```python
from build123d import *

# Parameters (mm, degrees)
BOSS_EXTRUDE1_DEPTH = 20
CUT_EXTRUDE1_REACH  = 38.702
SKETCH2_R           = 2.5
SKETCH5_W           = 10
SKETCH5_H           = 18
CUT_EXTRUDE4_DEPTH  = 54.272627403
SKETCH6_R           = 4
CUT_EXTRUDE5_DEPTH  = 46.762260698
SKETCH8_W           = 6
SKETCH8_H           = 22.840741565
CUT_EXTRUDE6_DEPTH  = 37.702076275
SKETCH12_W          = 3.539135452
SKETCH12_H          = 18
CUT_EXTRUDE7_DEPTH  = 41.024339686
CUT_EXTRUDE8_REACH  = 39.827
SKETCH13_W          = 12
SKETCH13_H          = 14.840741565
FILLET2_R           = 0.5


with BuildPart() as part:
    # Sketch1 → Boss-Extrude1 (new body)
    with BuildSketch(Plane.XY):
        Polygon((-3.287943452, 12.452372753), (-3.287943452, -24.388368812), (6.712056548, -24.388368812), (6.712056548, 17.547627247), (11.11006124, 19.788522565), (6.570156243, 28.698587807), (-7.827848449, 21.362437994), align=None)
    extrude(amount=BOSS_EXTRUDE1_DEPTH)

    # Sketch2 → Cut-Extrude1 (cut, up to next)
    with BuildSketch(Plane(origin=(0, 0, 0), x_dir=(-1, 0, 0), z_dir=(0, 0, -1)), mode=Mode.PRIVATE) as cut_extrude1_sk1:
        with Locations((-1.712056548, -19.388368812)):
            Circle(SKETCH2_R)
    cut_extrude1_tool1 = extrude(cut_extrude1_sk1.sketch, amount=-CUT_EXTRUDE1_REACH, mode=Mode.PRIVATE) & part.part
    # Sketch2 → Cut-Extrude1 (cut, up to next)
    with BuildSketch(Plane(origin=(0, 0, 0), x_dir=(-1, 0, 0), z_dir=(0, 0, -1)), mode=Mode.PRIVATE) as cut_extrude1_sk2:
        with Locations((-1.712056548, 20.611631188)):
            Circle(SKETCH2_R)
    cut_extrude1_tool2 = extrude(cut_extrude1_sk2.sketch, amount=-CUT_EXTRUDE1_REACH, mode=Mode.PRIVATE) & part.part
    add(cut_extrude1_tool1.solids().sort_by_distance((1.712057, -19.388369, 0))[0], mode=Mode.SUBTRACT)
    add(cut_extrude1_tool2.solids().sort_by_distance((1.712057, 20.611631, 0))[0], mode=Mode.SUBTRACT)

    # Sketch5 → Cut-Extrude4 (cut, through all)
    with BuildSketch(Plane(origin=(-10.254664976, 20.125913213, 0), x_dir=(0.891006524188368, 0.4539904997395467, 0), z_dir=(-0.4539904997395467, 0.891006524188368, 0))):
        with Locations((10.843123689, -10)):
            Rectangle(SKETCH5_W, SKETCH5_H)
    extrude(amount=-CUT_EXTRUDE4_DEPTH, mode=Mode.SUBTRACT)

    # Sketch6 → Cut-Extrude5 (cut, through all)
    with BuildSketch(Plane(origin=(16.824821219, 8.572674594, 0), x_dir=(0, 0, -1), z_dir=(0.891006524188368, 0.45399049973954647, 0))):
        with Locations(Location((-10, 17.587840455, 0), (0, 0, 90))):
            Circle(SKETCH6_R)
    extrude(amount=-CUT_EXTRUDE5_DEPTH, mode=Mode.SUBTRACT)

    # Sketch8 → Cut-Extrude6 (cut, through all)
    with BuildSketch(Plane.XY.offset(20)):
        with Locations((1.712056548, -2.96799803)):
            Rectangle(SKETCH8_W, SKETCH8_H)
    extrude(amount=-CUT_EXTRUDE6_DEPTH, mode=Mode.SUBTRACT)

    # Sketch12 → Cut-Extrude7 (cut, through all)
    with BuildSketch(Plane.XZ.offset(-8.452372753)):
        with Locations((0.481624274, 10)):
            Rectangle(SKETCH12_W, SKETCH12_H)
    extrude(amount=-CUT_EXTRUDE7_DEPTH, mode=Mode.SUBTRACT)

    # Sketch13 → Cut-Extrude8 (cut, up to next)
    with BuildSketch(Plane.ZY.offset(3.287943452), mode=Mode.PRIVATE) as cut_extrude8_sk1:
        with Locations((10, -6.96799803)):
            Rectangle(SKETCH13_W, SKETCH13_H)
    cut_extrude8_tool1 = extrude(cut_extrude8_sk1.sketch, amount=-CUT_EXTRUDE8_REACH, mode=Mode.PRIVATE) & part.part
    add(cut_extrude8_tool1.solids().sort_by_distance((-3.287943, -6.967998, 10))[0], mode=Mode.SUBTRACT)

    # Fillet2
    fillet2_edges = [part.edges().sort_by_distance(p)[0] for p in [
        (-2.287943452, -14.388368812, 4),
        (-1.287943452, -14.388368812, 18),
        (-1.287943452, -14.388368812, 2),
        (4.712056548, -14.388368812, 10),
        (-1.287943452, -6.96799803, 4),
        (-2.287943452, 0.452372753, 4),
        (-1.287943452, 0.452372753, 10),
        (-2.287943452, 0.452372753, 16),
        (-2.287943452, -14.388368812, 16),
        (-1.287943452, -6.96799803, 16),
        (1.712056548, 8.452372753, 19),
        (1.712056548, 8.452372753, 0),
        (1.712056548, 8.452372753, 1),
        (4.712056548, -2.96799803, 0),
        (-1.287943452, -2.96799803, 0),
        (1.712056548, -14.388368812, 0),
        (1.712056548, 8.452372753, 20),
        (4.712056548, -2.96799803, 20),
        (1.712056548, -14.388368812, 20),
        (-1.287943452, -2.96799803, 20),
        (-3.287943452, -14.388368812, 10),
        (-3.287943452, -6.96799803, 4),
        (-3.287943452, 0.452372753, 10),
        (-3.287943452, -6.96799803, 16),
        (1.712056548, -24.388368812, 20),
        (1.712056548, -24.388368812, 0),
        (-3.287943452, -24.388368812, 10),
        (-3.287943452, -5.96799803, 20),
        (-5.55789595, 16.907405373, 20),
        (-3.287943452, 12.452372753, 10),
        (-5.55789595, 16.907405373, 0),
        (-3.287943452, -5.96799803, 0),
        (-0.628846103, 25.030512901, 20),
        (-0.593371027, 25.048588355, 19),
        (-5.048403648, 22.778635856, 10),
        (-7.827848449, 21.362437994, 10),
        (-0.628846103, 25.030512901, 0),
        (-0.593371027, 25.048588355, 1),
        (3.861661594, 27.318540854, 10),
        (6.570156243, 28.698587807, 10),
        (8.840108742, 24.243555186, 20),
        (8.840108742, 24.243555186, 0),
        (11.11006124, 19.788522565, 10),
        (7.55681157, 17.97805143, 19),
        (8.911058894, 18.668074906, 20),
        (7.55681157, 17.97805143, 1),
        (8.401566592, 18.408475612, 10),
        (6.712056548, 8.622530187, 1),
        (4.712056548, 6.037513445, 19),
        (6.712056548, 8.622530187, 19),
        (4.712056548, 3.622654137, 10),
        (6.712056548, -0.302566874, 10),
        (8.911058894, 18.668074906, 0),
        (6.712056548, -3.420370782, 0),
        (6.712056548, -24.388368812, 10),
        (6.712056548, -3.420370782, 20),
    ]]
    fillet(fillet2_edges, radius=FILLET2_R - 0.0001)  # a hair under: the kernel refuses the full size


solid = part.part
```
Work out the finished part from the listing and answer in its coordinate system (mm). A direction names the side the tool comes from. Give positions to 0.01 mm unless a question says otherwise; leave off trailing zeros. Write each loop counter-clockwise with the first axis right and the second up, starting at its lowest first coordinate (ties: lowest second). Pieces come first, ordered by that corner, then holes. Notation, with made-up numbers: (69.5, 23) - (86.5, 23) arc R33 ccw to (86.5, 62) - close; hole circle Ø7 at (33, -15). An arc over 180 degrees is marked (long way). Use one line per item in the form item = value.
1. A cutting plane is placed at C-C (y = -16). Write down the section's boundary in (x, z), and give its area (3 significant figures).
Filled in:
outline = (-3.29, 0.5) arc R0.5 ccw to (-2.79, 0) - (6.21, 0) arc R0.5 ccw to (6.71, 0.5) - (6.71, 19.5) arc R0.5 ccw to (6.21, 20) - (-2.79, 20) arc R0.5 ccw to (-3.29, 19.5) - close
area = 200 mm^2
2. Determine the mould class of faces 5 (the face through (-2, -7, 16)), 6 (the face through (2, 10, 20)), 7 (the face through (9.978, 19.212, 9.867)) for opening direction Z: released by +Z, released by -Z, zero draft, split by the parting line, or undercut.
Filled in:
face_5 = undercut
face_6 = released by +Z
face_7 = zero draft
3. A cutting plane is placed at D-D (z = 11). State how many separate pieces and enclosed holes the cut face has, and give its area (3 significant figures).
Filled in:
separate_pieces = 5
enclosed_holes = 1
area = 149 mm^2
4. Consider L1, parallel to Z at x = 3, y = 24; L2, parallel to X at y = -8, z = 4.75; L3, parallel to X at y = 11, z = 14.25. Determine where each line is inside the solid, lowest interval first.
Filled in:
L1 = 0 to 1, 19 to 20
L2 = 4.71 to 6.71
L3 = -3.29 to -1.29
5. For faces 1 (the face through (5.65, 23.81, 14.13)), 2 (the face through (8.513, 18.634, 0.143)), 3 (the face through (6.712, -13, 10)), 4 (the face through (-2, 0.452, 10)), determine the directions among +Z, -Z, +X, -X, +Y, -Y from which every point of the face is accessible in a straight line to the end or side of a thin tool.
Filled in:
face_1 = none
face_2 = -Z, +X, -Y
face_3 = +Z, -Z, +X, -Y
face_4 = -X
6. A cutting plane is placed at B-B (y = -10.5). Write down the section's boundary in (x, z).
Filled in:
outline = (-3.29, 0.5) arc R0.5 ccw to (-2.79, 0) - (-1.79, 0) arc R0.5 ccw to (-1.29, 0.5) - (-1.29, 3.5) arc R0.5 ccw to (-1.79, 4) - (-2.79, 4) arc R0.5 ccw to (-3.29, 3.5) - close; (-3.29, 16.5) arc R0.5 ccw to (-2.79, 16) - (-1.79, 16) arc R0.5 ccw to (-1.29, 16.5) - (-1.29, 19.5) arc R0.5 ccw to (-1.79, 20) - (-2.79, 20) arc R0.5 ccw to (-3.29, 19.5) - close; (4.71, 0.5) arc R0.5 ccw to (5.21, 0) - (6.21, 0) arc R0.5 ccw to (6.71, 0.5) - (6.71, 19.5) arc R0.5 ccw to (6.21, 20) - (5.21, 20) arc R0.5 ccw to (4.71, 19.5) - close
7. Each of these flat-tipped pins is pushed along its axis until it touches: pin 1 Ø1 at (y, z) = (-11.5, 3) entering from +X; pin 2 Ø6 at (x, z) = (-5, 8) entering from +Y; pin 3 Ø4 at (x, y) = (1.71, -19.39) entering from +Z; pin 4 Ø9.5 at (y, z) = (-7.5, 10.5) entering from -X. Where does it stop, or does it pass through?
Filled in:
pin_1 = 6.71
pin_2 = 22.61
pin_3 = through
pin_4 = 4.71
8. A cutting plane is placed at A-A (z = 17). Write down the section's boundary in (x, y), and give its area (3 significant figures).
Filled in:
outline = (-7.6, 20.92) - (-3.34, 12.56) arc R0.5 cw to (-3.29, 12.33) - (-3.29, -23.89) arc R0.5 ccw to (-2.79, -24.39) - (6.21, -24.39) arc R0.5 ccw to (6.71, -23.89) - (6.71, -0.42) arc R0.5 ccw to (6.66, -0.2) - (5.66, 1.77) arc R0.5 ccw to (4.71, 1.54) - (4.71, -13.89) arc R0.5 cw to (4.21, -14.39) - (-0.79, -14.39) arc R0.5 cw to (-1.29, -13.89) - (-1.29, 15.4) - (-4.82, 22.33) arc R0.5 ccw to (-5.49, 22.55) - (-7.38, 21.59) arc R0.5 ccw to start; (4.09, 26.87) - (8.17, 18.85) arc R0.5 ccw to (8.85, 18.64) - (10.66, 19.56) arc R0.5 ccw to (10.88, 20.23) - (6.8, 28.25) arc R0.5 ccw to (6.12, 28.47) - (4.31, 27.55) arc R0.5 ccw to start; hole circle Ø5 at (1.71, -19.39)
area = 227 mm^2
